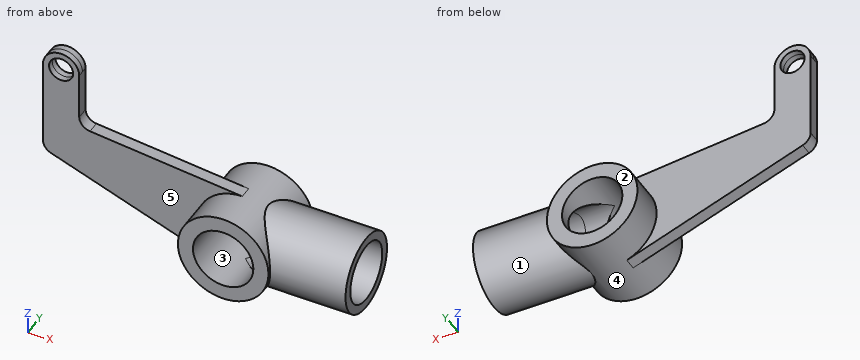
from build123d import *

# Parameters (mm, degrees)
SKETCH_1_R          = 37.5
SKETCH_1_R_2        = 25
EXTRUDE_1_DEPTH     = 70
SKETCH_2_R          = 32.5
SKETCH_2_R_2        = 25
EXTRUDE_2_DEPTH     = 100
CUT_EXTRUDE_START   = -100
SKETCH_3_R          = 25
CUT_EXTRUDE_1_DEPTH = 100
SKETCH_4_R          = 25
CUT_EXTRUDE_2_DEPTH = 100
EXTRUDE_START       = 35
SKETCH_5_R          = 15
SKETCH_5_R_2        = 10
EXTRUDE_3_DEPTH     = 5
FILLET_2_R          = 10


with BuildPart() as part:
    # 草圖1 → 填料-伸長1 (new body)
    with BuildSketch(Plane(origin=(0, 0, 0), x_dir=(1, 0, 0), z_dir=(0, 1, 0))):
        with Locations(Location((0, 0, 0), (0, 0, 270))):
            Circle(SKETCH_1_R)
        with Locations(Location((0, 0, 0), (0, 0, 270))):
            Circle(SKETCH_1_R_2, mode=Mode.SUBTRACT)
    extrude(amount=EXTRUDE_1_DEPTH)

    # 草圖2 → 填料-伸長2 (add)
    with BuildSketch(Plane(origin=(0, 0, 0), x_dir=(0, 0, -1), z_dir=(1, 0, 0))):
        with Locations(Location((0, 35, 0), (0, 0, 180))):
            Circle(SKETCH_2_R)
        with Locations(Location((0, 35, 0), (0, 0, 180))):
            Circle(SKETCH_2_R_2, mode=Mode.SUBTRACT)
    extrude(amount=EXTRUDE_2_DEPTH)

    # 草圖3 → 除料-伸長1 (cut)
    with BuildSketch(Plane(origin=(0, 70, 0), x_dir=(1, 0, 0), z_dir=(0, 1, 0)).offset(CUT_EXTRUDE_START)):
        with Locations(Location((0, 0, 0), (0, 0, 270))):
            Circle(SKETCH_3_R)
    extrude(amount=CUT_EXTRUDE_1_DEPTH, mode=Mode.SUBTRACT)

    # 草圖4 → 除料-伸長2 (cut)
    with BuildSketch(Plane(origin=(100, 0, 0), x_dir=(0, 0, -1), z_dir=(1, 0, 0)).offset(CUT_EXTRUDE_START)):
        with Locations((0, 35)):
            Circle(SKETCH_4_R)
    extrude(amount=CUT_EXTRUDE_2_DEPTH, mode=Mode.SUBTRACT)

    # 草圖5 → 填料-伸長3 (add, symmetric)
    # profile 1 of 2: a face of its own
    with BuildSketch(Plane(origin=(0, 0, 0), x_dir=(1, 0, 0), z_dir=(0, 1, 0)).offset(EXTRUDE_START)):
        with BuildLine():
            ThreePointArc((0, -37.5), (-36.930290738, -6.511806663), (-12.825755375, 35.238473279))
            Line((-12.825755375, 35.238473279), (-165, -20.148422186))
            Line((-165, -20.148422186), (-165, -100))
            ThreePointArc((-165, -100), (-150, -85), (-135, -100))
            Line((-135, -100), (-135, -51.689071761))
            Line((-135, -51.689071761), (0, -37.5))
        make_face()
    # profile 2 of 2: a face of its own
    with BuildSketch(Plane(origin=(0, 0, 0), x_dir=(1, 0, 0), z_dir=(0, 1, 0)).offset(EXTRUDE_START)):
        with Locations((-150, -100)):
            Circle(SKETCH_5_R)
        with Locations(Location((-150, -100, 0), (0, 0, 270))):
            Circle(SKETCH_5_R_2, mode=Mode.SUBTRACT)
    extrude(amount=EXTRUDE_3_DEPTH, both=True)

    # 圓角2
    fillet_2_edges = [part.edges().sort_by_distance(p)[0] for p in [
        (-165, 35, 20.148422186),
        (-135, 35, 51.689071761),
    ]]
    fillet(fillet_2_edges, radius=FILLET_2_R)


solid = part.part
Geometry: final body of the model. Coordinates: model frame, mm. Face numbers are marked on the shaded views. A direction names the side the tool comes from. Coordinates: 2 decimals unless noted, no trailing zeros. Loops run counter-clockwise (first coordinate to the right, second up) from the corner with the lowest first, then second, coordinate; pieces in that order, holes last. Notation, with made-up numbers: (40.5, -33.75) - (88.5, -33.75) arc R17 cw to (88.5, -22.75) - close; hole circle Ø11 at (-22, 65.5). An arc over 180 degrees is marked (long way). One line per question, with ' | ' between items. Start each with the question number.
(1) Cut plane C-C on y = 20. Output: boundary loops of the cut face in (x, z).
(2) Cut plane D-D on x = 65. Output: boundary loops of the cut face in (y, z), and give its area (3 significant figures).
(3) Cut plane A-A on z = 93.5. Output: boundary loops of the cut face in (x, y), and give its area (3 significant figures).
(4) First-contact query: pin 1 (12 mm diameter, centred on x = 59.5, z = 17, fed in from +Y); pin 2 (1 mm diameter, centred on x = -74, z = 4, fed in from +Y); pin 3 (6 mm diameter, centred on y = 41, z = 61, fed in from -X); pin 4 (16 mm diameter, centred on x = -150, z = 100, fed in from +Y). Flat tips, straight axial feed; report the tip coordinate or a pass-through.
(5) Reachability of the marked faces 1 and 2 from +Z, -Z, +X, -X, +Y, -Y: full face, straight path, thin tool, end or side. Return the list, or none.
(6) Draft query along X for the marked faces 3, 4 and 5. Return one class per face: +X half, -X half, draft (parallel to the pull), parting line (faces both ways), or undercut.
(7) Ray query, L1, parallel to Z at x = 33, y = 23; L2, parallel to Y at x = -43, z = 37; L3, parallel to Z at x = 15.5, y = 29.5. Return the intervals inside material, ascending. Write a range as from..to.
(8) Cut plane B-B on x = 14. Output: boundary loops of the cut face in (y, z), and give its area (3 significant figures).
Here are the results:
1) outline: (15, -20) arc R25 cw (long way) to (15, 20) - (100, 20) - (100, 28.83) - (23.98, 28.83) arc R37.5 ccw (long way) to (23.98, -28.83) - (100, -28.83) - (100, -20) - close
2) outline: circle Ø65 at (35, 0); hole circle Ø50 at (35, 0) | area: 1,350 mm²
3) outline: (-165, 30) - (-157.6, 30) - (-157.6, 40) - (-165, 40) - close; (-142.4, 30) - (-135, 30) - (-135, 40) - (-142.4, 40) - close | area: 148 mm²
4) pin 1: y = 65.58 | pin 2: y = 40 | pin 3: x = -165 | pin 4: through
5) face 1: +X | face 2: +Z, -Z, +X, -X, +Y
6) face 3: undercut | face 4: parting line | face 5: draft
7) L1: -30.2..-21.93, 21.93..30.2 | L2: 30..40 | L3: -34.15..-24.39, 24.39..34.15
8) outline: (0, -34.79) - (70, -34.79) - (70, -20.71) - (49, -20.71) arc R25 cw to (21, -20.71) - (0, -20.71) - close; (0, 20.71) - (21, 20.71) arc R25 cw to (49, 20.71) - (70, 20.71) - (70, 34.79) - (0, 34.79) - close | area: 1,810 mm²
